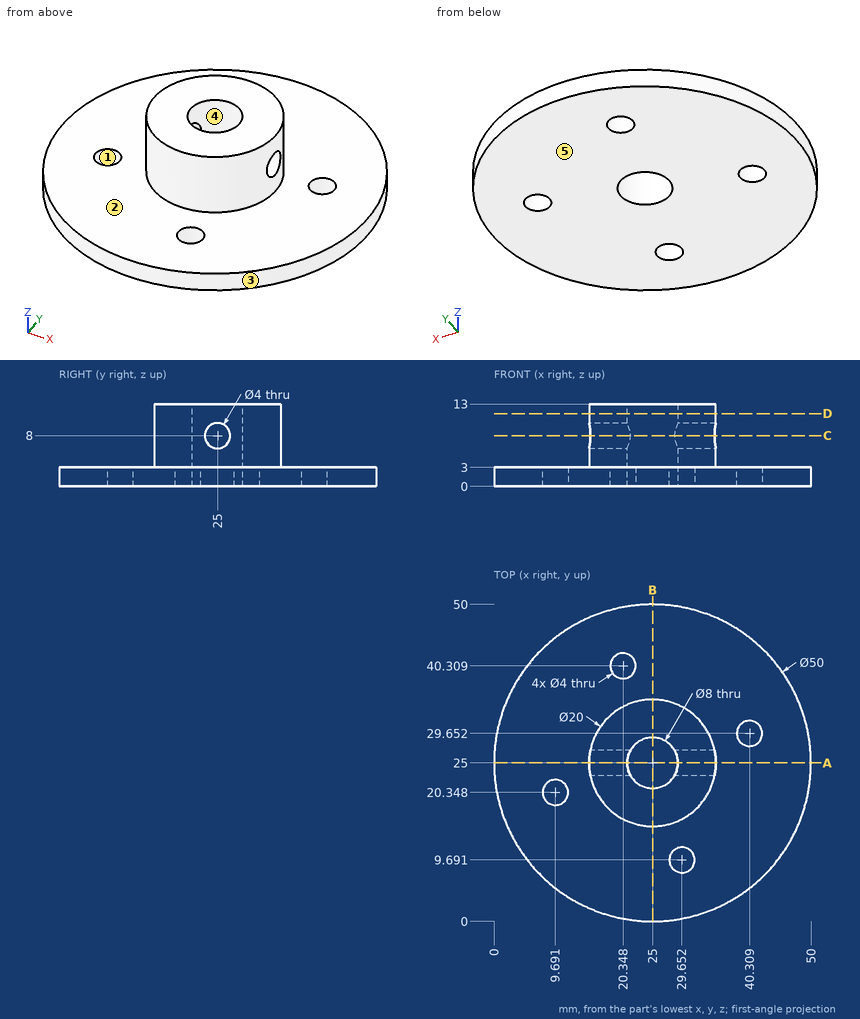
Job drawing, mm, ordinate dimensions from the low corner. One solid piece. A direction names the side the tool comes from. Give positions to 0.01 mm unless a question says otherwise; leave off trailing zeros. Write each loop counter-clockwise with the first axis right and the second up, starting at its lowest first coordinate (ties: lowest second). Pieces come first, ordered by that corner, then holes. Notation, with made-up numbers: (-36.75, -25) - (-12.75, -25) arc R22 cw to (-12.75, -18) - close; hole circle Ø11 at (29.25, -22.75). An arc over 180 degrees is marked (long way). Answer as CSV lines item,"result".
1. 3-axis set-ups, long thin cutter, end or side, ignore diameter. For the marked faces 1 and 2: which of +Z, -Z, +X, -X, +Y, -Y reach the whole face in a straight line?
Responses:
face 1,"+Z, -Z"
face 2,"+Z"
2. Band-saw the part on C-C (z = 8). Write the cut outline in (x, y), and give its area (3 significant figures).
Responses:
outline,"(15.2, 23) arc R10 ccw to (34.8, 23) - (28.46, 23) arc R4 cw to (21.54, 23) - close; (15.2, 27) - (21.54, 27) arc R4 cw to (28.46, 27) - (34.8, 27) arc R10 ccw to start"
area,"215 mm2"
3. Band-saw the part on D-D (z = 11.5). Write the cut outline in (x, y).
Responses:
outline,"circle Ø20 at (25, 25); hole circle Ø8 at (25, 25)"
4. Band-saw the part on B-B (x = 25). Write the cut outline in (y, z).
Responses:
outline,"(0, 0) - (21, 0) - (21, 13) - (15, 13) - (15, 3) - (0, 3) - close; (29, 0) - (50, 0) - (50, 3) - (35, 3) - (35, 13) - (29, 13) - close"
5. Band-saw the part on A-A (y = 25). Write the cut outline in (x, z).
Responses:
outline,"(0, 0) - (21, 0) - (21, 6) - (15, 6) - (15, 3) - (0, 3) - close; (15, 10) - (21, 10) - (21, 13) - (15, 13) - close; (29, 0) - (50, 0) - (50, 3) - (35, 3) - (35, 6) - (29, 6) - close; (29, 10) - (35, 10) - (35, 13) - (29, 13) - close"
6. Drill centre lines: L1, parallel to Y at x = 25, z = 5.25; L2, parallel to X at y = 27.5, z = 12.25; L3, parallel to Z at x = 46, y = 35.5. Where is each one in solid material? Low to high. Write a range as [from, to].
Responses:
L1,"y = [15, 21], [29, 35]"
L2,"x = [15.32, 21.88], [28.12, 34.68]"
L3,"z = [0, 3]"
7. Pin check, flat tips, straight feed: pin 1 (6.5 mm diameter, centred on x = 29.65, y = 9.69, fed in from +Z); pin 2 (6 mm diameter, centred on y = 6, z = 2, fed in from -X); pin 3 (3 mm diameter, centred on y = 14, z = 4, fed in from -X). Stop position of each tip, or through.
Responses:
pin 1,"stops at z = 3"
pin 2,"stops at x = 5.79"
pin 3,"stops at x = 2.04"
8. Two-plate mould, pull along Y, no slides. Class the marked faces 3, 4 and 5: +Y half, -Y half, draft (parallel to the pull), parting line (faces both ways), or undercut.
Responses:
face 3,"parting line"
face 4,"undercut"
face 5,"draft"
